Autodesk Inventor part; units mm, degrees
ref_plane "YZ Plane" through (0, 0, 0) normal (1, 0, 0) x (0, 1, 0)
ref_plane "XZ Plane" through (0, 0, 0) normal (0, 1, 0) x (-1, 0, 0)
ref_plane "XY Plane" through (0, 0, 0) normal (0, 0, 1) x (1, 0, 0)
sketch "草圖1" plane through (0, 0, 0) normal (0, 0, 1) x (1, 0, 0)
  line L0 (0, 0) -> (80, 0)
  line L1 (80, 0) -> (80, 8)
  line L2 (60, 8) -> (0, 8)
  line L3 (0, 8) -> (0, 0)
  line L4 (80, 8) -> (60, 8)
  line L5 (60, 8) -> (60, 15)
  line L6 (60, 15) -> (80, 15)
  line L7 (80, 15) -> (80, 8)
  dimension "d0" = 80
  dimension "d1" = 20
  dimension "d2" = 15
  dimension "d3" = 8
extrude "擠出1" add sketch "草圖1" along normal mid plane 20
sketch "草圖2" plane through (0, 0, 0) normal (0, 0, 1) x (1, 0, 0)
  line L0 (70, 31.4394) -> (70, 6.5)
  line L1 (60, 15) -> (80, 15)
  line L2 (80, 0) -> (80, 15)
  arc A0 (70, 6.5) -> (70, 21.5) centre (70, 14) ccw
  line L3 (70, 14) -> (77.5, 14)
  point P0 (0, 0)
  dimension "d14" = 7.5
  dimension "d16" = 10
  dimension "d56" = 1
sketch "草圖3" plane through (0, 8, -10) normal (0, 1, 0) x (1, 0, 0)
  line L0 (60, 0) -> (60, -20)
  line L1 (0, 0) -> (60, 0)
  line L2 (60, 0) -> (60, -5)
  line L3 (60, -5) -> (0, -5)
  line L4 (0, -5) -> (0, 0)
  line L5 (0, -20) -> (60, -20)
  line L6 (60, -20) -> (60, -15)
  line L7 (60, -15) -> (0, -15)
  line L8 (0, -15) -> (0, -20)
  line L9 (60, -20) -> (0, -20)
  point P0 (0, -10)
  dimension "d10" = 5
  dimension "d11" = 5
extrude "擠出2" cut sketch "草圖3" against normal blind 20
revolve "迴轉2" cut sketch "草圖2" angle 360 about axis through (70, 31.4394, 0) along (0, -1, 0)
sketch "草圖4" plane through (0, 8, 5) normal (0, 1, 0) x (1, 0, 0)
  line L0 (12, 8) -> (19, 8)
  line L1 (19, 8) -> (19, 2)
  line L2 (19, 2) -> (12, 2)
  line L3 (12, 2) -> (12, 8)
  point P0 (0, 5)
  dimension "d34" = 3
  dimension "d35" = 6
  dimension "d36" = 7
  dimension "d37" = 12
extrude "擠出3" add sketch "草圖4" along normal blind 11
sketch "草圖7" plane through (12, 8, 3) normal (0, 0, 1) x (1, 0, 0)
  circle A0 centre (3.5, 8) radius 2
  line L0 (7, 0) -> (0, 0)
  line L1 (7, 0) -> (7, 11)
  line L2 (0, 11) -> (7, 11)
  line L3 (0, 0) -> (0, 11)
  point P0 (-12, -8)
  dimension "d38" = 3.5
  dimension "d39" = 4
  dimension "d40" = 3
extrude "擠出6" cut sketch "草圖7" against normal blind 10 contours A0
fillet "圓角3" radius 2 2 edges at (12, 19, 0) (19, 19, 0)
fillet "圓角2" radius 3 2 edges at (0, 8, 0) (0, 0, 0)
sketch "草圖6" plane through (60, 0, 5) normal (0, 0, 1) x (1, 0, 0)
  arc A0 (-57, 8) -> (-60, 5) centre (-57, 5) ccw
  arc A1 (-60, 3) -> (-57, 0) centre (-57, 3) ccw
  circle A2 centre (-56, 4) radius 2
  line L0 (-57, 8) -> (0, 8)
  line L1 (-60, 3) -> (-60, 5)
  point P0 (-60, 0)
  dimension "d29" = 4
  dimension "d30" = 4
  dimension "d31" = 4
extrude "擠出5" cut sketch "草圖6" against normal through all
sketch "草圖10" plane through (0, 0, -10) normal (0, 0, -1) x (-1, 0, 0)
  circle A0 centre (-70, 16) radius 7.5
  line L0 (-60, 15) -> (-80, 15)
  point P0 (0, 0)
  dimension "d52" = 15
  dimension "d53" = 1
extrude "擠出9" cut sketch "草圖10" against normal blind 8
properties part number "連趕2"
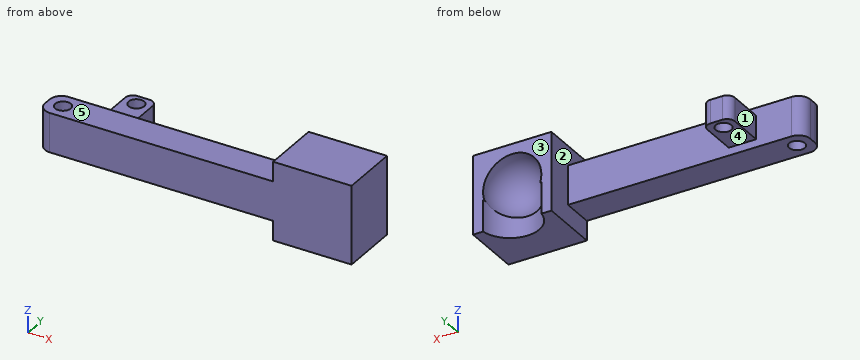
Build history of the part. All positions in model axes, mm. Face numbers are marked on the shaded views. A direction names the side the tool comes from. Round coordinates to 2 decimals unless told otherwise and drop trailing zeros. Loops run counter-clockwise (first coordinate to the right, second up) from the corner with the lowest first, then second, coordinate; pieces in that order, holes last. Notation, with made-up numbers: (42, 54.5) -> (72, 54.5) arc R26 ccw to (72, 87.5) -> close; hole circle Ø5 at (-8.5, 6.5). An arc over 180 degrees is marked (long way). One line per item, written item: value. Start each with the question number.
Q1. 3-axis set-ups, long thin cutter, end or side, ignore diameter. For the marked faces 1, 2, 3, 4 and 5: which of +Z, -Z, +X, -X, +Y, -Y reach the whole face in a straight line?
Q2. Cut at A-A on y = 4. List the corners of the cut face in (x, z).
Q3. Drop flat-ended pins along their axis: pin 1 Ø3 at (x, z) = (43.5, 0.5) entering from +Y; pin 2 Ø6.5 at (y, z) = (13.5, -1) entering from -X; pin 3 Ø4 at (x, y) = (37.5, 5) entering from -Z; pin 4 Ø3.5 at (x, y) = (15.5, 16) entering from +Z. Give the stop position or say it passes through.
Q4. Cut at B-B on x = 4. List the corners of the cut face in (y, z).
Q5. Cut at C-C on z = -7.5. List the corners of the cut face in (x, y), plus the area to 3 significant figures.
Q6. Probe line 1 along X through (y, z) = (12.25, 1.5); line 2 along Y through (x, z) = (4, 1); line 3 along X through (y, z) = (10.25, 1.75) (3 decimals). List the from-to ranges inside material, lowest first.
Q7. Cut at D-D on z = 1.75. List the corners of the cut face in (x, y).
Computed:
1. face 1: +Z, -Z, -X, +Y
1. face 2: +Y
1. face 3: +Z, -Z, +X, +Y
1. face 4: -Z, -X, +Y
1. face 5: +Z, -X, +Y, -Y
2. outline: (0, -5) -> (2, -5) -> (2, 5) -> (0, 5) -> close; (6, -5) -> (60, -5) -> (60, -10) -> (80, -10) -> (80, 10) -> (60, 10) -> (60, 5) -> (6, 5) -> close
3. pin 1: y = 8
3. pin 2: x = 12
3. pin 3: z = -5
3. pin 4: through
4. outline: (0, -5) -> (2, -5) -> (2, 5) -> (0, 5) -> close; (6, -5) -> (8, -5) -> (8, 5) -> (6, 5) -> close
5. outline: (60, 0) -> (80, 0) -> (80, 15) -> (77.43, 15) arc R7.5 cw to (62.57, 15) -> (60, 15) -> close
5. area: 227 mm²
6. line 1: 12 to 19, 60 to 62.86, 77.14 to 80
6. line 2: 0 to 2, 6 to 8
6. line 3: 12 to 19, 60 to 63.745, 76.255 to 80
7. outline: (0, 3) arc R3 ccw to (3, 0) -> (80, 0) -> (80, 15) -> (77.22, 15) arc R7.29 cw (long way) to (62.78, 15) -> (60, 15) -> (60, 8) -> (19, 8) -> (19, 17) arc R2 ccw to (17, 19) -> (14, 19) arc R2 ccw to (12, 17) -> (12, 8) -> (3, 8) arc R3 ccw to (0, 5) -> close; hole circle Ø4 at (4, 4); hole circle Ø4 at (15.5, 16)
